The model under review builds one solid part; all positions refer to its coordinate system, in mm. A direction names the side the tool comes from. Coordinates: 2 decimals unless noted, no trailing zeros. Loops run counter-clockwise (first coordinate to the right, second up) from the corner with the lowest first, then second, coordinate; pieces in that order, holes last. Notation, with made-up numbers: (89, 67.25) - (126, 67.25) arc R34 ccw to (126, 97.25) - close; hole circle Ø5 at (61, 50). An arc over 180 degrees is marked (long way). Answer in a Markdown table with one row per item. Add a question column.
(1) Mouldability with a two-part tool opening along X and no side actions: class faces 6 (the flat face through (-8, 1, -15.575)), 7 (the flat face through (3, 11, -33.019)), 8 (the cylindrical face through (7.602, -1.103, -14.009)), 9 (the cylindrical face through (14.578, -1.329, 21.648)) as +X half, -X half, draft (parallel to the pull), parting line (faces both ways), or undercut.
(2) We need section C-C on z = 18. Write out the cut boundary in (x, y).
(3) Machinability: for faces 1 (the cylindrical face through (10.25, -1.69, -24.42)), 2 (the cylindrical face through (-7.74, 18.38, -4.02)), 3 (the flat face through (-10, 7, 33.019)), 4 (the cylindrical face through (7.602, -1.103, 13.964)), 5 (the cylindrical face through (10.25, -1.69, 24.17)), which of the approach directions +Z, -Z, +X, -X, +Y, -Y give a long, thin tool a straight path to every point of the face, cutting with its end or side? Answer none if there is none.
(4) For line 1 along Z through (x, y) = (0, 20.25); line 2 along Y through (x, z) = (0, -22); line 3 along X through (y, z) = (-0.5, 24), list the stretches that pass through material, from the lowest coordinate up.
(5) We need section B-B on x = 1. Give the number of separate pieces and of enclosed holes in the cut face, plus the area to 3 significant figures.
(6) For P1, Ø8, axis at y = 15, z = 7, coming from the +X side; P2, Ø10.5, axis at x = -3, y = 1.5, coming from the +Z side (3 decimals); P3, Ø10.5, axis at x = -2.5, y = 1.5, coming from the -Z side (3 decimals); P4, Ø2, axis at x = -6.5, y = -13, coming from the -Z side, all flat-tipped, find the tip position at first contact; note any pin that passes through.
(7) We need section A-A on y = -6.5. Write out the cut boundary in (x, z) (3 decimals).
(8) We need section D-D on x = -9.5. Write out the cut boundary in (y, z) (3 decimals), plus the area to 3 significant figures.
from build123d import *

# Parameters (mm, degrees)
SCALE1_SCALE = 0.623


with BuildPart() as part:
    # Sketch2 → RevolveBody (revolve)
    with BuildSketch(Plane(origin=(0, 0, 0), x_dir=(0, 0, -1), z_dir=(1, 0, 0))):
        with BuildLine():
            Line((53, 23.6), (15.977797095, 23.6))
            ThreePointArc((15.977797095, 23.6), (0, 28.5), (-15.977797095, 23.6))
            Line((-15.977797095, 23.6), (-53, 23.6))
            Line((-53, 23.6), (-53, 0))
            Line((-53, 0), (53, 0))
            Line((53, 0), (53, 23.6))
        make_face()
    revolve(axis=Axis((0, 0, 97.71293904), (0, 0, -1)))

    # Sketch3 → RevStem (revolve)
    with BuildSketch(Plane(origin=(0, 0, 0), x_dir=(0, 0, -1), z_dir=(1, 0, 0))):
        with BuildLine():
            Line((19, 38), (19, 21.242645786))
            ThreePointArc((19, 21.242645786), (10.169429559, 26.62391223), (0, 28.5))
            Line((0, 28.5), (0, 38))
            Line((0, 38), (19, 38))
        make_face()
    revolve(axis=Axis((0, 38, 0), (0, -1, 0)))

    # Sketch4 → CoreBody (revolve, cut)
    with BuildSketch(Plane(origin=(0, 0, 0), x_dir=(0, 0, -1), z_dir=(1, 0, 0))):
        Polygon((53, 16.85), (53, 0), (-53, 0), (-53, 16.85), (-25, 16.85), (-25, 12.5), (25, 12.5), (25, 16.85), align=None)
    revolve(axis=Axis((0, 0, -53), (0, 0, 1)), mode=Mode.SUBTRACT)

    # Sketch5 → CoreStem (revolve, cut)
    with BuildSketch(Plane(origin=(0, 0, 0), x_dir=(0, 0, -1), z_dir=(1, 0, 0))):
        with BuildLine():
            Line((14, 38), (0, 38))
            Line((0, 38), (0, -23.5))
            ThreePointArc((0, -23.5), (22.313704008, -7.37215121), (14, 18.874586088))
            Line((14, 18.874586088), (14, 38))
        make_face()
    revolve(axis=Axis((0, 58.20350065, 0), (0, -1, 0)), mode=Mode.SUBTRACT)


with BuildPart() as part_1:
    # Scale1: scaled about (-8.85e-07, 1.551247427, 4.25e-06)
    add(part.part.scale(SCALE1_SCALE).moved(Location((-3.34e-07, 0.58482028, 1.602e-06))))


solid = part_1.part
Outcome:
| question | item | result |
|---|---|---|
| 1 | face 6 | undercut |
| 1 | face 7 | draft |
| 1 | face 8 | undercut |
| 1 | face 9 | parting line |
| 2 | outline | circle Ø29.41 at (0, 0.58); hole circle Ø21 at (0, 0.58) |
| 3 | face 1 | -Z |
| 3 | face 2 | +Y |
| 3 | face 3 | +Z, +X, -X, +Y, -Y |
| 3 | face 4 | +Z, -Z |
| 3 | face 5 | +Z |
| 4 | line 1 | -11.84 to -8.72, 8.72 to 11.84 |
| 4 | line 2 | -14.12 to -9.91, 11.08 to 15.29 |
| 4 | line 3 | -14.66 to -10.44, 10.44 to 14.66 |
| 5 | separate pieces | 3 |
| 5 | enclosed holes | 0 |
| 5 | area | 567 mm² |
| 6 | P1 | x = 13.06 |
| 6 | P2 | z = 15.575 |
| 6 | P3 | z = -15.575 |
| 6 | P4 | z = -33.02 |
| 7 | outline | (-12.883, -33.019) - (-7.746, -33.019) - (-7.746, -15.575) - (-3.233, -15.575) - (-3.233, -12.398) arc R12.812 cw to (-3.233, 12.398) - (-3.233, 15.575) - (-7.746, 15.575) - (-7.746, 33.019) - (-12.883, 33.019) - (-12.883, 9.954) arc R16.281 ccw to (-12.883, -9.954) - close; (3.233, -15.575) - (7.746, -15.575) - (7.746, -33.019) - (12.883, -33.019) - (12.883, -9.954) arc R16.281 ccw to (12.883, 9.954) - (12.883, 33.019) - (7.746, 33.019) - (7.746, 15.575) - (3.233, 15.575) - (3.233, 12.398) arc R12.812 cw to (3.233, -12.398) - close |
| 8 | outline | (-10.637, -33.019) - (-3.882, -33.019) - (-3.882, -15.575) - (5.051, -15.575) - (5.051, -33.019) - (11.806, -33.019) - (11.806, -9.954) arc R15 ccw to (13.819, -7.061) - (24.259, -7.061) - (24.259, 7.061) - (13.819, 7.061) arc R15 ccw to (11.806, 9.954) - (11.806, 33.019) - (5.051, 33.019) - (5.051, 15.575) - (-3.882, 15.575) - (-3.882, 33.019) - (-10.637, 33.019) - (-10.637, 9.954) arc R15 ccw to (-10.637, -9.954) - close; hole circle Ø22.28 at (0.585, 0) |
| 8 | area | 1,010 mm² |
